from build123d import *

# Parameters (mm, degrees)
SKETCH1_W                                            = 90
SKETCH1_H                                            = 85
BOSS_EXTRUDE1_DEPTH                                  = 6
F_4_6_4_6_DIAMETER_HOLE1_D                           = 4.6
BOSS_EXTRUDE2_DEPTH                                  = 85
CSK_FOR_M4_HEX_SOCKET_COUNTERSUNK_HEAD_S_D           = 4.8
CSK_FOR_M4_HEX_SOCKET_COUNTERSUNK_HEAD_S_CSINK_D     = 9.18
CSK_FOR_M4_HEX_SOCKET_COUNTERSUNK_HEAD_S_CSINK_ANGLE = 90
CUT_EXTRUDE1_DEPTH                                   = 20
CUT_EXTRUDE2_START                                   = -65
CUT_EXTRUDE2_DEPTH                                   = 20


with BuildPart() as part:
    # Sketch1 → Boss-Extrude1 (new body)
    with BuildSketch(Plane(origin=(0, 0, 0), x_dir=(1, 0, 0), z_dir=(0, 1, 0))):
        with Locations((45, 42.5)):
            Rectangle(SKETCH1_W, SKETCH1_H)
    extrude(amount=BOSS_EXTRUDE1_DEPTH)

    # Ø4.6 (4.6) Diameter Hole1 (through all)
    with Locations(Plane(origin=(0, 6, 0), x_dir=(1, 0, 0), z_dir=(0, 1, 0))):
        with Locations((75.310889132, 60), (45, 7.5), (14.689110868, 60)):
            Hole(F_4_6_4_6_DIAMETER_HOLE1_D / 2)

    # Sketch8 → Boss-Extrude2 (add)
    with BuildSketch(Plane.XY):
        Polygon((5, 12), (11, 6), (0, 6), (-12, 6), (-12, 12), align=None)
        Polygon((79, 6), (90, 6), (102, 6), (102, 12), (85, 12), align=None)
    extrude(amount=-BOSS_EXTRUDE2_DEPTH)

    # CSK for M4 Hex Socket Countersunk Head Screw1 (through all)
    with Locations(Plane(origin=(0, 12, 0), x_dir=(1, 0, 0), z_dir=(0, 1, 0))):
        with Locations((-6, 10), (-6, 75), (96, 75), (96, 10), (-6, 30), (-6, 55), (96, 55), (96, 30)):
            CounterSinkHole(CSK_FOR_M4_HEX_SOCKET_COUNTERSUNK_HEAD_S_D / 2, CSK_FOR_M4_HEX_SOCKET_COUNTERSUNK_HEAD_S_CSINK_D / 2, counter_sink_angle=CSK_FOR_M4_HEX_SOCKET_COUNTERSUNK_HEAD_S_CSINK_ANGLE)

    # Sketch16 → Cut-Extrude1 (cut)
    with BuildSketch(Plane(origin=(0, 0, -10), x_dir=(0, 1, 0), z_dir=(0, 0, 1))):
        Polygon((6, 8.4), (6, 3.6), (9.81, 3.6), (12, 1.41), (26, 24.59), (9.81, 8.4), align=None)
        Polygon((12, -91.41), (26, -114.59), (9.81, -98.4), (6, -98.4), (6, -93.6), (9.81, -93.6), align=None)
    extrude(amount=-CUT_EXTRUDE1_DEPTH, mode=Mode.SUBTRACT)

    # Sketch16<4> → Cut-Extrude2 (cut)
    with BuildSketch(Plane(origin=(0, 0, -10), x_dir=(0, 1, 0), z_dir=(0, 0, 1)).offset(CUT_EXTRUDE2_START)):
        Polygon((6, 8.4), (6, 3.6), (9.81, 3.6), (12, 1.41), (26, 24.59), (9.81, 8.4), align=None)
        Polygon((26, -114.59), (9.81, -98.4), (6, -98.4), (6, -93.6), (9.81, -93.6), (12, -91.41), align=None)
    extrude(amount=CUT_EXTRUDE2_DEPTH, mode=Mode.SUBTRACT)


solid = part.part
Can you work these out from the model? Positions are in its coordinate system, mm. A direction names the side the tool comes from. Coordinates: 2 decimals unless noted, no trailing zeros. Write each loop counter-clockwise with the first axis right and the second up, starting at its lowest first coordinate (ties: lowest second). Pieces come first, ordered by that corner, then holes. Notation, with made-up numbers: (-7, -30) - (5, -30) arc R24 cw to (5, -11) - close; hole circle Ø9 at (5.5, 28.25). An arc over 180 degrees is marked (long way). Return JSON: item names as keys, results as strings. Group by question number.
Item 1: If we section it at B-B (x = -6): Write out the boundary of the cut face in (y, z), then the cut area to 3 significant figures.
Item 2: If we section it at D-D (y = 3): Write out the boundary of the cut face in (x, z), then the cut area to 3 significant figures.
Item 3: We'd pull the mould along X, two halves only. Please class faces 4 (the face through (46, 5, 0)), 5 (the face through (102, 9, -42)), 6 (the face through (98.4, 8, -20)): pulls with the +X half, pulls with the -X half, needs draft (parallel to the pull), parting line crosses it, or undercut.
Item 4: If we section it at A-A (y = 8): Write out the boundary of the cut face in (x, z).
Item 5: Please list where these lines run through material, in increasing order: probe 1 along X at (y, z) = (1.6, -60); probe 2 along X at (y, z) = (10.5, -20); probe 3 along Z at (x, y) = (96, 6.25).
Item 6: Which directions (+Z, -Z, +X, -X, +Y, -Y) give clear straight access to the entire face, cutting with the end or side of a thin tool? Please do faces 1 (the face through (45, 6, -43)), 2 (the face through (96.06, 10.16, -7.25)), 3 (the face through (96.05, 7.88, -52.6)).
Item 7: If we section it at C-C (z = -28): Write out the boundary of the cut face in (x, y), then the cut area to 3 significant figures.
Item 8: I'm going to push flat-ended pins straight in: pin 1 Ø6.5 at (y, z) = (2, -45) entering from +X; pin 2 Ø6 at (x, z) = (94, -47) entering from -Y; pin 3 Ø5 at (x, z) = (72.5, -42.5) entering from +Y; pin 4 Ø3.5 at (x, z) = (14.69, -60) entering from -Y. Where does each tip first touch, or does it pass through?
Return value:
{
 "1": {"outline": "(6, -85) - (12, -85) - (12, -79.59) - (9.81, -77.4) - (6, -77.4) - close; (6, -52.6) - (9.81, -52.6) - (12, -50.41) - (12, -34.59) - (9.81, -32.4) - (6, -32.4) - close; (6, -7.6) - (9.81, -7.6) - (12, -5.41) - (12, 0) - (6, 0) - close", "area": "203 mm^2"},
 "2": {"outline": "(0, -85) - (90, -85) - (90, 0) - (0, 0) - close; hole circle Ø4.6 at (14.69, -60); hole circle Ø4.6 at (45, -7.5); hole circle Ø4.6 at (75.31, -60)", "area": "7,600 mm^2"},
 "3": {"face 4": "needs draft", "face 5": "pulls with the +X half", "face 6": "undercut"},
 "4": {"outline": "(-12, -85) - (9, -85) - (9, 0) - (-12, 0) - close; (81, -85) - (102, -85) - (102, 0) - (81, 0) - close; hole (-8.4, -75) arc R2.4 ccw to (-3.6, -75) - (-3.6, -55) arc R2.4 ccw to (-8.4, -55) - close; hole (-8.4, -30) arc R2.4 ccw to (-3.6, -30) - (-3.6, -10) arc R2.4 ccw to (-8.4, -10) - close; hole (93.6, -75) arc R2.4 ccw to (98.4, -75) - (98.4, -55) arc R2.4 ccw to (93.6, -55) - close; hole (93.6, -30) arc R2.4 ccw to (98.4, -30) - (98.4, -10) arc R2.4 ccw to (93.6, -10) - close"},
 "5": {"probe 1": "x = 0 to 12.39, 16.99 to 73.01, 77.61 to 90", "probe 2": "x = -12 to -9.09, -2.91 to 6.5, 83.5 to 92.91, 99.09 to 102", "probe 3": "z = -85 to -77.4, -52.6 to -32.4, -7.6 to 0"},
 "6": {"face 1": "+Z, -Z, +Y", "face 2": "+Y", "face 3": "+Y, -Y"},
 "7": {"outline": "(-12, 6) - (-8.4, 6) - (-8.4, 9.81) - (-10.59, 12) - (-12, 12) - close; (-3.6, 6) - (0, 6) - (0, 0) - (90, 0) - (90, 6) - (93.6, 6) - (93.6, 9.81) - (91.41, 12) - (85, 12) - (79, 6) - (11, 6) - (5, 12) - (-1.41, 12) - (-3.6, 9.81) - close; (98.4, 6) - (102, 6) - (102, 12) - (100.59, 12) - (98.4, 9.81) - close", "area": "713 mm^2"},
 "8": {"pin 1": "stops at x = 90", "pin 2": "stops at y = 6", "pin 3": "stops at y = 6", "pin 4": "passes through"}
}
